Build history of the part. All positions in model axes, mm. A direction names the side the tool comes from. Give positions to 0.01 mm unless a question says otherwise; leave off trailing zeros. Use a Markdown table: item, result.
Autodesk Inventor part; units mm, degrees
ref_plane "РабПлоскость1" through (0, 0, 0) normal (0, 1, 0) x (-1, 0, 0)
ref_plane "YZ Plane" through (0, 0, 0) normal (1, 0, 0) x (0, 1, 0)
ref_plane "XY Plane" through (0, 0, 0) normal (0, 0, 1) x (1, 0, 0)
sketch "Эскиз1" plane through (0, 0, 0) normal (0, 0, 1) x (1, 0, 0)
  circle A0 centre (0, 0) radius 5
  dimension "d0" = 10
extrude "Выдавливание1" add sketch "Эскиз1" along normal blind 80
sketch "Эскиз2" plane through (0, 0, 0) normal (0, 0, -1) x (-1, 0, 0)
  line L0 (0, 0) -> (0, 3)
  line L1 (0, 3) -> (-4, 3)
  circle A0 centre (0, 0) radius 5
  line L2 (4, 3) -> (0, 3)
extrude "Выдавливание2" cut sketch "Эскиз2" against normal blind 10 contours L1 A0 L2 picked at (-2.4012, 3.2796)
ref_plane "РабПлоскость1" through (0, 0, 0) normal (0, 1, 0) x (-1, 0, 0)
sketch "Эскиз3" plane through (0, 0, 0) normal (0, 1, 0) x (-1, 0, 0)
  line L0 (0, 10) -> (0, 80)
  line L1 (5, 80) -> (-5, 80)
  line L2 (0, 10) -> (0, 15)
  line L3 (0, 15) -> (6, 15)
  line L4 (0, 15) -> (0, 20)
  line L5 (0, 20) -> (4, 20)
  line L6 (0, 20) -> (0, 45)
  line L7 (0, 45) -> (0, 70)
  line L8 (0, 70) -> (4, 70)
  line L9 (0, 70) -> (0, 75)
  line L10 (0, 75) -> (6, 75)
  line L11 (0, 45) -> (6, 45)
  spline S0 degree 4 poles (0, 80) (13.7387, 74.1571) (-5.0029, 77.0727) (17.394, 45) (-5.0029, 12.9273) (13.7387, 15.8429) (0, 10) knots 0 0 0 0 0 0.409508 0.590492 1 1 1 1 1
  point P0 (0, 0)
  dimension "d7" = 5
  dimension "d8" = 6
  dimension "d9" = 5
  dimension "d10" = 4
  dimension "d11" = 25
  dimension "d12" = 25
  dimension "d13" = 4
revolve "Вращение1" add sketch "Эскиз3" angle 360 about axis through (0, 0, 10) along (0, 0, 1)
properties part number "Рукаядь рукоядки"
1) Wall check: line 1 (Y direction, x = 3, z = 20.5); line 2 (Y direction, x = 3, z = 9); line 3 (Z direction, x = 0.5, y = 3.5). Give the ranges that are in metal, low to high. Write a range as from..to.
Computed:
| item | result |
|---|---|
| line 1 | y = -4..4 |
| line 2 | y = -4..3 |
| line 3 | z = 10..80 |
2) Tool access for faces 1 (the flat face through (0, 0, 80)), 2 (the flat face through (0, 4, 10)), 3 (the cylindrical face through (-0.651, -4.957, 6.186)), 4 (the cylindrical face through (-1.08, 4.88, 78.71)): list every direction of +Z, -Z, +X, -X, +Y, -Y with a clear straight run to the whole face (end or side of a thin tool).
Computed:
| item | result |
|---|---|
| face 1 | +Z, +X, -X, +Y, -Y |
| face 2 | -Z, +X, -X, +Y |
| face 3 | -Z |
| face 4 | +Z |
3) Pin check, flat tips, straight feed: P1, Ø0.6, axis at x = -1, y = 4, coming from the -Z side; P2, Ø5, axis at x = -2.5, z = 49.5, coming from the +Y side; P3, Ø2, axis at y = -3.5, z = 60.5, coming from the +X side. Stop position of each tip, or through.
Computed:
| item | result |
|---|---|
| P1 | stops at z = 10 |
| P2 | stops at y = 5.9 |
| P3 | stops at x = 4.33 |
4) Two-plate mould, pull along Z, no slides. Class faces 5 (the cylindrical face through (-1.08, 4.88, 64.34)), 6 (the flat face through (0, -1, 0)), 7 (the flat face through (0, 3, 5)), 8 (the cylindrical face through (4.77, -1.5, 25.42)): +Z half, -Z half, draft (parallel to the pull), parting line (faces both ways), or undercut.
Computed:
| item | result |
|---|---|
| face 5 | undercut |
| face 6 | -Z half |
| face 7 | draft |
| face 8 | undercut |
